Can you work these out from the model? Positions are in its coordinate system, mm. A direction names the side the tool comes from. Round coordinates to 2 decimals unless told otherwise and drop trailing zeros. Write each loop counter-clockwise with the first axis right and the second up, starting at its lowest first coordinate (ties: lowest second). Pieces come first, ordered by that corner, then holes. Notation, with made-up numbers: M 87.5,26 L 100.5,26 A36 ccw 100.5,61 Z; hole C 56,70.25 d11. An arc over 180 degrees is marked long. Answer as a JSON object with one key per item and string values. Group by question number.
1) Please list where these lines run through material, in increasing order: L1, parallel to Y at x = 90, z = 98; L2, parallel to Z at x = -17, y = 4.75; L3, parallel to Y at x = 32, z = -58. Write a range as [from, to].
2) On a 3-axis mill with a long thin cutter (end or side, diameter ignored), from which of +Z, -Z, +X, -X, +Y, -Y can I reach the whole of each face in a straight line? I mean faces 1 (the flat face through (100, 2, 11)), 2 (the flat face through (-1, 3, 1)), 3 (the flat face through (-1, 3, -108)). Say none if no direction works.
3) I'm going to push flat-ended pins straight in: pin 1 Ø1.5 at (x, z) = (-49.5, 4) entering from +Y; pin 2 Ø4.5 at (x, z) = (-30, -107.5) entering from -Y; pin 3 Ø1 at (x, y) = (-15.5, 6.5) entering from +Z. Where does each tip first touch, or does it pass through?
4) Suppose I cut it at A-A, the plane x = 78.5. Write out the boundary of the cut face in (y, z).
5) Suppose I cut it at B-B, the plane z = 85. Write out the boundary of the cut face in (x, y), and give its area (3 significant figures).
6) If we mould it in two halves opening along Z, with no side actions, what happens to faces 4 (the flat face through (-1, 10, 96.5)), 5 (the flat face through (-1, 6, -103)), 6 (the flat face through (-1, 10, 99.5))? For each: +Z half, -Z half, draft (parallel to the pull), parting line (faces both ways), or undercut.
from build123d import *

# Parameters (mm, degrees)
SKETCH1_W           = 200
SKETCH1_H           = 205
BOSS_EXTRUDE1_DEPTH = 3
SKETCH2_W           = 200
SKETCH2_H           = 20
BOSS_EXTRUDE2_DEPTH = 3
CUT_EXTRUDE1_REACH  = 152.639
SKETCH3_R           = 2
LPATTERN1_COUNT     = 4
LPATTERN1_PITCH     = 60
SKETCH4_W           = 200
SKETCH4_H           = 3
BOSS_EXTRUDE3_DEPTH = 15
CUT_EXTRUDE2_REACH  = 237.091
SKETCH5_R           = 1.5
LPATTERN2_COUNT     = 4
LPATTERN2_PITCH     = 60


with BuildPart() as part:
    # Sketch1 → Boss-Extrude1 (new body)
    with BuildSketch(Plane(origin=(0, 0, 0), x_dir=(1, 0, 0), z_dir=(0, 1, 0))):
        Rectangle(SKETCH1_W, SKETCH1_H)
    extrude(amount=BOSS_EXTRUDE1_DEPTH)

    # Sketch2 → Boss-Extrude2 (add)
    with BuildSketch(Plane(origin=(0, 3, 0), x_dir=(1, 0, 0), z_dir=(0, 1, 0))):
        with Locations((0, 102.5)):
            Rectangle(SKETCH2_W, SKETCH2_H)
    extrude(amount=BOSS_EXTRUDE2_DEPTH)

    # Sketch3 → Cut-Extrude1 (cut, up to next)
    with BuildSketch(Plane(origin=(0, 6, 0), x_dir=(1, 0, 0), z_dir=(0, 1, 0)), mode=Mode.PRIVATE) as cut_extrude1_sk1:
        with Locations(Location((-90, 107.5, 0), (0, 0, 270))):
            Circle(SKETCH3_R)
    cut_extrude1_tool1 = extrude(cut_extrude1_sk1.sketch, amount=-CUT_EXTRUDE1_REACH, mode=Mode.PRIVATE) & part.part
    cut_extrude1 = cut_extrude1_tool1.solids().sort_by_distance((-90, 6, -107.5))[0]
    add(cut_extrude1, mode=Mode.SUBTRACT)

    # LPattern1: Cut-Extrude1 ×4
    with Locations(*[(i * LPATTERN1_PITCH, 0, 0) for i in range(1, LPATTERN1_COUNT)]):
        add(cut_extrude1, mode=Mode.SUBTRACT)

    # Sketch4 → Boss-Extrude3 (add)
    with BuildSketch(Plane(origin=(0, 3, 0), x_dir=(1, 0, 0), z_dir=(0, 1, 0))):
        with Locations((0, -98)):
            Rectangle(SKETCH4_W, SKETCH4_H)
    extrude(amount=BOSS_EXTRUDE3_DEPTH)

    # Sketch5 → Cut-Extrude2 (cut, up to next)
    with BuildSketch(Plane.XY.offset(99.5), mode=Mode.PRIVATE) as cut_extrude2_sk1:
        with Locations((-90, 10.5)):
            Circle(SKETCH5_R)
    cut_extrude2_tool1 = extrude(cut_extrude2_sk1.sketch, amount=-CUT_EXTRUDE2_REACH, mode=Mode.PRIVATE) & part.part
    cut_extrude2 = cut_extrude2_tool1.solids().sort_by_distance((-90, 10.5, 99.5))[0]
    add(cut_extrude2, mode=Mode.SUBTRACT)

    # LPattern2: Cut-Extrude2 ×4
    with Locations(*[(i * LPATTERN2_PITCH, 0, 0) for i in range(1, LPATTERN2_COUNT)]):
        add(cut_extrude2, mode=Mode.SUBTRACT)


solid = part.part
Results:
{
 "1": {"L1": "[0, 9], [12, 18]", "L2": "[-112.5, -92.5], [96.5, 99.5]", "L3": "[0, 3]"},
 "2": {"face 1": "+Z, -Z, +X, +Y, -Y", "face 2": "+X, -X, +Y", "face 3": "-Z, +X, -X, -Y"},
 "3": {"pin 1": "y = 3", "pin 2": "y = 3", "pin 3": "z = 99.5"},
 "4": {"outline": "M 0,-102.5 L 3,-102.5 L 3,-112.5 L 6,-112.5 L 6,-92.5 L 3,-92.5 L 3,96.5 L 18,96.5 L 18,99.5 L 3,99.5 L 3,102.5 L 0,102.5 Z"},
 "5": {"outline": "M -100,0 L 100,0 L 100,3 L -100,3 Z", "area": "600 mm^2"},
 "6": {"face 4": "undercut", "face 5": "draft", "face 6": "+Z half"}
}
